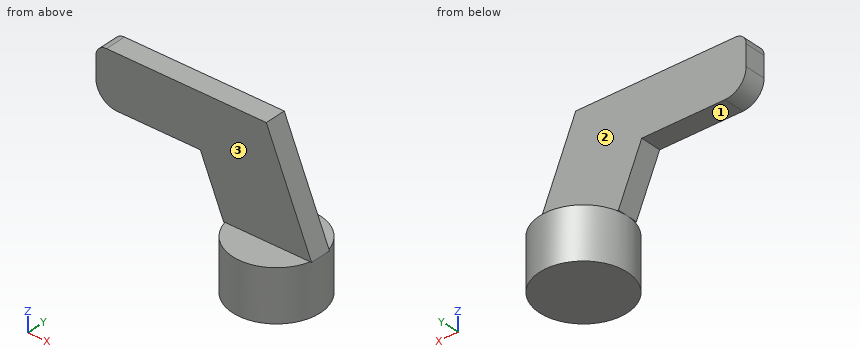
from build123d import *

# Parameters (mm, degrees)
F1_DEPTH = 6.35
F2_R     = 26.3416
F3_DEPTH = 30.734


with BuildPart() as f1:
    # F0 (on Front) → F1 (new body, symmetric)
    with BuildSketch(Plane.XZ):
        with BuildLine():
            Line((-24.249891, 0), (28.433308, 0))
            Line((28.433308, 0), (1.333008, 64.996654))
            Line((1.333008, 64.996654), (-94.431851, 64.996654))
            ThreePointArc((-94.431851, 64.996654), (-98.921979, 63.136782), (-100.781851, 58.646654))
            Line((-100.781851, 58.646654), (-100.781851, 46.1244))
            ThreePointArc((-100.781851, 46.1244), (-97.062107, 37.144144), (-88.081851, 33.4244))
            Line((-88.081851, 33.4244), (-38.186166, 33.4244))
            Line((-38.186166, 33.4244), (-24.249891, 0))
        make_face()
    extrude(amount=F1_DEPTH, both=True)

    # F2 (on Top) → F3 (join)
    with BuildSketch(Plane.XY):
        with Locations((2.091708, 0)):
            Circle(F2_R)
    extrude(amount=-F3_DEPTH)


solid = f1.part
For this review, take the finished solid that the model builds, in its own axes (mm). Face numbers are marked on the shaded views. A direction names the side the tool comes from. Give positions to 0.01 mm unless a question says otherwise; leave off trailing zeros. Loops run counter-clockwise (first coordinate to the right, second up) from the corner with the lowest first, then second, coordinate; pieces in that order, holes last. Notation, with made-up numbers: M 66,-17 L 74,-17 A34 cw 74,20 Z; hole C 79,12 d10. An arc over 180 degrees is marked long. Put each result on its own line as item: value. Start each with the question number.
(1) Add section A-A, the plane x = -18.5. Write out the cut boundary in (y, z).
(2) Wall thickness on L1, parallel to Y at x = 6, z = 48.5; L2, parallel to Z at x = 19.5, y = -18: over which ranges is each line inside the solid? List them lowest first.
(3) Add section C-C, the plane y = 8. Write out the cut boundary in (x, z), then the cut area to 3 significant figures.
(4) Add section B-B, the plane z = -20.5. Write out the cut boundary in (x, y), then the cut area to 3 significant figures.
(5) For pin 1 (10 mm diameter, centred on x = -34, z = 42.5, fed in from +Y); pin 2 (4 mm diameter, centred on x = -65, y = 1, fed in from -Z); pin 3 (1.5 mm diameter, centred on x = -75, z = 31.5, fed in from -Y); pin 4 (4 mm diameter, centred on y = 7.5, z = -8.5, fed in from +X), all flat-tipped, find the tip position at first contact; note any pin that passes through.
(6) Add section D-D, the plane x = -45. Write out the cut boundary in (y, z), then the cut area to 3 significant figures.
(7) Machinability: for the marked faces 1, 2 and 3, which of the approach directions +Z, -Z, +X, -X, +Y, -Y give a long, thin tool a straight path to every point of the face, cutting with its end or side? Answer none if there is none.
Result:
1. outline: M -16.43,-30.73 L 16.43,-30.73 L 16.43,0 L 6.35,0 L 6.35,65 L -6.35,65 L -6.35,0 L -16.43,0 Z
2. L1: y = -6.35 to 6.35
2. L2: z = -30.73 to 0
3. outline: M -23.01,-30.73 L 27.19,-30.73 L 27.19,0 L -23.01,0 Z
3. area: 1,540 mm^2
4. outline: C 2.09,0 d52.68
4. area: 2,180 mm^2
5. pin 1: stops at y = 6.35
5. pin 2: stops at z = 33.42
5. pin 3: passes through
5. pin 4: stops at x = 27.85
6. outline: M -6.35,33.42 L 6.35,33.42 L 6.35,65 L -6.35,65 Z
6. area: 401 mm^2
7. face 1: -Z, -X, +Y, -Y
7. face 2: +Z, +X, -X, +Y
7. face 3: +Z, +X, -X, -Y
